Build history of the part. All positions in model axes, mm. Face numbers are marked on the shaded views. A direction names the side the tool comes from. Give positions to 0.01 mm unless a question says otherwise; leave off trailing zeros. Loops run counter-clockwise (first coordinate to the right, second up) from the corner with the lowest first, then second, coordinate; pieces in that order, holes last. Notation, with made-up numbers: (13, 37.5) -> (65, 37.5) arc R31 cw to (65, 71.5) -> close; hole circle Ø6 at (-1, 59). An arc over 180 degrees is marked (long way). One line per question, with ' | ' between items. Start each with the question number.
(1) 3-axis set-ups, long thin cutter, end or side, ignore diameter. For the marked faces 1, 2 and 3: which of +Z, -Z, +X, -X, +Y, -Y reach the whole face in a straight line?
(2) Slice it at B-B, the plane z = 1.65. Write the cut outline in (x, y).
(3) Drill centre lines: L1, parallel to Y at x = 4, z = 1.4; L2, parallel to X at y = -4.5, z = 1.7; L3, parallel to Y at x = 10.25, z = 2. Where is each one in solid material? Low to high. Write a range as from..to.
(4) Flat gauge pins, fed straight in: pin 1 Ø0.8 at (y, z) = (-9.5, 1.5) entering from +X; pin 2 Ø3 at (x, y) = (4, 10.6) entering from +Z; pin 3 Ø0.8 at (x, z) = (10.5, 1) entering from -Y; pin 4 Ø1 at (y, z) = (9, 2) entering from -X. Where does each tip first touch, or does it go through?
(5) Slice it at C-C, the plane y = 10.6. Write the cut outline in (x, z), then the cut area to 3 significant figures.
(6) Mould opens along Y. For the marked faces 4, 5 and 6 say: pulls with the +Y half, pulls with the -Y half, needs draft (parallel to the pull), parting line crosses it, or undercut.
(7) Slice it at A-A, the plane x = 4. Write the cut outline in (y, z), then the cut area to 3 significant figures.
(8) Slice it at D-D, the plane x = 14.5. Write the cut outline in (y, z).
```python
from build123d import *

# Parameters (mm, degrees)
ESQUISSE1_R        = 1.75
BOSS_EXTRU_1_DEPTH = 3


with BuildPart() as part:
    # Esquisse1 → Boss.-Extru.1 (new body)
    with BuildSketch(Plane.XY):
        with BuildLine():
            Line((3.177327772, 17), (17, 17))
            Line((17, 17), (17, 15))
            Line((17, 15), (11, 15))
            ThreePointArc((11, 15), (9.585786438, 14.414213562), (9, 13))
            Line((9, 13), (9, -2))
            ThreePointArc((9, -2), (9.292893219, -2.707106781), (10, -3))
            Line((10, -3), (11.55, -3))
            Line((11.55, -3), (11.55, -8))
            Line((11.55, -8), (10, -8))
            ThreePointArc((10, -8), (9.292893219, -8.292893219), (9, -9))
            Line((9, -9), (9, -10))
            Line((9, -10), (3.5, -10))
            ThreePointArc((3.5, -10), (2.792893219, -9.707106781), (2.5, -9))
            Line((2.5, -9), (2.5, -1))
            ThreePointArc((2.5, -1), (2.498565392, -0.946454153), (2.494265684, -0.89306194))
            Line((2.494265684, -0.89306194), (1, 13))
            ThreePointArc((1, 13), (1.463823787, 15.340120425), (3.177327772, 17))
        make_face()
        with Locations((4, 10.6)):
            Circle(ESQUISSE1_R, mode=Mode.SUBTRACT)
    extrude(amount=BOSS_EXTRU_1_DEPTH)


solid = part.part
```
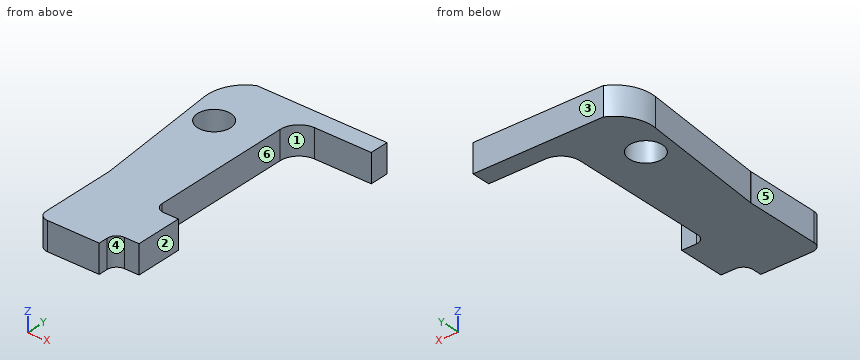
Final values:
1) face 1: +Z, -Z, +X | face 2: +Z, -Z, +X, -Y | face 3: +Z, -Z, +X, -X, +Y
2) outline: (1, 13) -> (2.49, -0.89) arc R1 cw to (2.5, -1) -> (2.5, -9) arc R1 ccw to (3.5, -10) -> (9, -10) -> (9, -9) arc R1 cw to (10, -8) -> (11.55, -8) -> (11.55, -3) -> (10, -3) arc R1 cw to (9, -2) -> (9, 13) arc R2 cw to (11, 15) -> (17, 15) -> (17, 17) -> (3.18, 17) arc R4 ccw to start; hole circle Ø3.5 at (4, 10.6)
3) L1: -10..8.85, 12.35..17 | L2: 2.5..11.55 | L3: -8..-3, 14.85..17
4) pin 1: x = 9 | pin 2: through | pin 3: y = -8 | pin 4: x = 1.38
5) outline: (1.26, 0) -> (2.25, 0) -> (2.25, 3) -> (1.26, 3) -> close; (5.75, 0) -> (9, 0) -> (9, 3) -> (5.75, 3) -> close | area: 12.7 mm2
6) face 4: pulls with the -Y half | face 5: needs draft | face 6: undercut
7) outline: (-10, 0) -> (8.85, 0) -> (8.85, 3) -> (-10, 3) -> close; (12.35, 0) -> (17, 0) -> (17, 3) -> (12.35, 3) -> close | area: 70.5 mm2
8) outline: (15, 0) -> (17, 0) -> (17, 3) -> (15, 3) -> close
